from build123d import *

# Parameters (mm, degrees)
BOSS_EXTRUDE1_DEPTH = 5.334


with BuildPart() as part:
    # Sketch1 → Boss-Extrude1 (new body)
    with BuildSketch(Plane.XY):
        with BuildLine():
            ThreePointArc((29.104915692, 69.046424835), (0, 74.93), (-29.104915692, 69.046424835))
            ThreePointArc((-29.104915692, 69.046424835), (-30.750210185, 62.710204346), (-26.565512441, 57.676022304))
            ThreePointArc((-26.565512441, 57.676022304), (0, 63.5), (26.565512441, 57.676022304))
            ThreePointArc((26.565512441, 57.676022304), (30.750210185, 62.710204346), (29.104915692, 69.046424835))
        make_face()
        Polygon((-17.78, 62.373825791), (-14.605, 64.206912895), (-14.605, 67.873087105), (-17.78, 69.706174209), (-20.955, 67.873087105), (-20.955, 64.206912895), align=None, mode=Mode.SUBTRACT)
        Polygon((17.78, 62.373825791), (20.955, 64.206912895), (20.955, 67.873087105), (17.78, 69.706174209), (14.605, 67.873087105), (14.605, 64.206912895), align=None, mode=Mode.SUBTRACT)
    extrude(amount=BOSS_EXTRUDE1_DEPTH)


solid = part.part
The listing builds one solid part. Answer for the finished solid, in the listing's coordinates (mm). A direction names the side the tool comes from. Give positions to 0.01 mm unless a question says otherwise; leave off trailing zeros. Loops run counter-clockwise (first coordinate to the right, second up) from the corner with the lowest first, then second, coordinate; pieces in that order, holes last. Notation, with made-up numbers: (61.25, 83.5) - (106.25, 83.5) arc R14 ccw to (106.25, 87.5) - close; hole circle Ø8 at (27.25, 15.25). An arc over 180 degrees is marked (long way). Answer as a JSON object with one key per item and string values.
1. A cutting plane is placed at B-B (z = 0.95). Write down the section's boundary in (x, y) (3 decimals).
Determined:
{"outline": "(-29.105, 69.046) arc R7.174 ccw to (-26.566, 57.676) arc R63.5 cw to (26.566, 57.676) arc R7.174 ccw to (29.105, 69.046) arc R74.93 ccw to start; hole (-20.955, 64.207) - (-17.78, 62.374) - (-14.605, 64.207) - (-14.605, 67.873) - (-17.78, 69.706) - (-20.955, 67.873) - close; hole (14.605, 64.207) - (17.78, 62.374) - (20.955, 64.207) - (20.955, 67.873) - (17.78, 69.706) - (14.605, 67.873) - close"}
2. Flat-ended cylindrical pins translate along their axes: pin 1 Ø1 at (x, z) = (6.5, 3) entering from +Y; pin 2 Ø3 at (x, z) = (-20, 3) entering from -Y; pin 3 Ø3 at (y, z) = (67, 3) entering from -X. Find the tip coordinate at first contact, or state that the pin passes through.
Determined:
{"pin 1": "y = 74.69", "pin 2": "y = 59.75", "pin 3": "x = -30.82"}
3. For a pull along Y with two mould halves and no side action, classify faces 3 (the flat face through (-19.39, 63.303, 2.63)), 4 (the flat face through (0, 66, 5.334)), 5 (the cylindrical face through (30.73, 62.62, 2.63)) as pulls with the +Y half, pulls with the -Y half, needs draft (parallel to the pull), parting line crosses it, or undercut.
Determined:
{"face 3": "undercut", "face 4": "needs draft", "face 5": "parting line crosses it"}
4. A cutting plane is placed at C-C (y = 59). Write down the section's boundary in (x, z).
Determined:
{"outline": "(-28.61, 0) - (-23.48, 0) - (-23.48, 5.33) - (-28.61, 5.33) - close; (23.48, 0) - (28.61, 0) - (28.61, 5.33) - (23.48, 5.33) - close"}
5. A cutting plane is placed at A-A (y = 64.75). Write down the section's boundary in (x, z) (3 decimals), then the cut area to 3 significant figures.
Determined:
{"outline": "(-30.907, 0) - (-20.955, 0) - (-20.955, 5.334) - (-30.907, 5.334) - close; (-14.605, 0) - (14.605, 0) - (14.605, 5.334) - (-14.605, 5.334) - close; (20.955, 0) - (30.907, 0) - (30.907, 5.334) - (20.955, 5.334) - close", "area": "262 mm²"}
6. A cutting plane is placed at D-D (x = -25). Write down the section's boundary in (y, z), then the cut area to 3 significant figures.
Determined:
{"outline": "(58.37, 0) - (70.64, 0) - (70.64, 5.33) - (58.37, 5.33) - close", "area": "65.4 mm²"}
7. For faces 1 (the cylindrical face through (-0.4, 63.5, 2.6)), 2 (the flat face through (-19, 69, 3)), determine the directions among +Z, -Z, +X, -X, +Y, -Y from which every point of the face is accessible in a straight line to the end or side of a thin tool.
Determined:
{"face 1": "+Z, -Z, -Y", "face 2": "+Z, -Z"}
8. Find the intervals of material crossed by L1, parallel to X at y = 64.5, z = 0.8 (3 decimals); L2, parallel to X at y = 69, z = 2.9; L3, parallel to Y at x = 16, z = 2.2, in increasing order. Write a range as [from, to].
Determined:
{"L1": "[-30.919, -20.955], [-14.605, 14.605], [20.955, 30.919]", "L2": "[-29.15, -19], [-16.56, 16.56], [19, 29.15]", "L3": "[61.45, 63.4], [68.68, 73.2]"}
